Source: CAD feature listing. Evaluate the final solid. Frame: model axes, mm. A direction names the side the tool comes from. Round coordinates to 2 decimals unless told otherwise and drop trailing zeros. Order: outer loops, then holes, each group sorted by start corner. A loop starts at its lowest first (then second) coordinate and runs counter-clockwise, first axis right, second up. Notation, with made-up numbers: (-27.75, 1) -> (-16.75, 1) arc R23 cw to (-16.75, 22) -> close; hole circle Ø9 at (62, 32). An arc over 180 degrees is marked (long way). Answer as CSV lines item,"result".
from build123d import *

# Parameters (mm, degrees)
SKETCH1_R           = 1.5
BOSS_EXTRUDE1_DEPTH = 2
BOSS_EXTRUDE2_DEPTH = 38.1
BOSS_EXTRUDE3_DEPTH = 1.5
BOSS_EXTRUDE6_DEPTH = 27.94


with BuildPart() as part:
    # Sketch1 → Boss-Extrude1 (new body)
    with BuildSketch(Plane(origin=(0, 0, 0), x_dir=(1, 0, 0), z_dir=(0, 1, 0))):
        Polygon((-14, -7.1960018), (-3.6637, -7.1960018), (-3.6637, -14.7), (-1.6637, -14.7), (-1.6637, -2), (1.6637, -2), (1.6637, -14.7), (3.6637, -14.7), (3.6637, -7.1960018), (14, -7.1960018), (14, 5.5039982), (-14, 5.5039982), align=None)
        with Locations(Location((-11, -0.8460018, 0), (0, 0, 270))):
            Circle(SKETCH1_R, mode=Mode.SUBTRACT)
        with Locations(Location((11, -0.8460018, 0), (0, 0, 270))):
            Circle(SKETCH1_R, mode=Mode.SUBTRACT)
    extrude(amount=BOSS_EXTRUDE1_DEPTH)

    # Sketch1_3 → Boss-Extrude2 (add)
    with BuildSketch(Plane(origin=(0, 0, 0), x_dir=(1, 0, 0), z_dir=(0, 1, 0))):
        Polygon((3.6637, 0), (-3.6637, 0), (-3.6637, -7.1960018), (-3.6637, -14.7), (-1.6637, -14.7), (-1.6637, -2), (1.6637, -2), (1.6637, -14.7), (3.6637, -14.7), (3.6637, -7.1960018), align=None)
    extrude(amount=BOSS_EXTRUDE2_DEPTH)

    # Sketch2 → Boss-Extrude3 (add)
    with BuildSketch(Plane(origin=(0, 0, 7.1960018), x_dir=(-1, 0, 0), z_dir=(0, 0, -1))):
        Polygon((3.6637, 2), (3.6637, 33.75), (14, 2), align=None)
        Polygon((-14, 2), (-3.6637, 2), (-3.6637, 33.75), align=None)
    extrude(amount=BOSS_EXTRUDE3_DEPTH)

    # Sketch6 → Boss-Extrude6 (add)
    with BuildSketch(Plane(origin=(0, 38.1, 0), x_dir=(1, 0, 0), z_dir=(0, 1, 0))):
        Polygon((1.6637, -14.7), (3.6637, -14.7), (3.6637, 0), (-3.6637, 0), (-3.6637, -14.7), (-1.6637, -14.7), (-1.6637, -2), (1.6637, -2), align=None)
    extrude(amount=BOSS_EXTRUDE6_DEPTH)

    # Mirror6: part across plane


with BuildPart() as part_1:
    add(part.part)
    add(part.part.mirror(Plane(origin=(0, 66.04, 0), x_dir=(0, 0, 1), z_dir=(0, -1, 0))))


solid = part_1.part
1. Reachability of faces 4 (the flat face through (-8, 10, 7.196)), 5 (the flat face through (1.664, 67, 8)), 6 (the flat face through (3.664, 67, 7)), 7 (the flat face through (0, 67, 0)) from +Z, -Z, +X, -X, +Y, -Y: full face, straight path, thin tool, end or side. Return the list, or none.
Results below:
face 4,"+Z, -X, +Y, -Y"
face 5,"+Z, +Y, -Y"
face 6,"+X"
face 7,"-Z, +X, -X"
2. Section query D-D on z = 12.5. Return loops of the section in (x, y).
Results below:
outline,"(-3.66, 0) -> (-1.66, 0) -> (-1.66, 132.08) -> (-3.66, 132.08) -> close; (1.66, 0) -> (3.66, 0) -> (3.66, 132.08) -> (1.66, 132.08) -> close"
3. Section query A-A on z = -2.5. Return loops of the section in (x, y), and give its area (3 significant figures).
Results below:
outline,"(-14, 0) -> (14, 0) -> (14, 2) -> (-14, 2) -> close; (-14, 130.08) -> (14, 130.08) -> (14, 132.08) -> (-14, 132.08) -> close"
area,"112 mm2"
4. Mould query, pull axis Y, two halves, no side actions, for faces 1 (the flat face through (8.76, 113.98, 6.46)), 2 (the flat face through (0, 0, 0)), 3 (the flat face through (0, 67, 2)). Classes: released by +Y, released by -Y, zero draft, split by the parting line, or undercut.
Results below:
face 1,"undercut"
face 2,"released by -Y"
face 3,"zero draft"
5. Pin query (flat end, axial travel): pin 1 (3 mm diameter, centred on x = -11, y = 14, fed in from +Z); pin 2 (2.5 mm diameter, centred on x = 11, z = 0.85, fed in from -Y); pin 3 (4 mm diameter, centred on x = 4.5, z = 5, fed in from -Y); pin 4 (10 mm diameter, centred on y = 46, z = 1, fed in from +X). Return the tip coordinate at first contact, or that it passes through.
Results below:
pin 1,"z = 7.2"
pin 2,"through"
pin 3,"y = 0"
pin 4,"x = 3.66"
6. Section query B-B on y = 87. Return loops of the section in (x, z).
Results below:
outline,"(-3.66, 0) -> (3.66, 0) -> (3.66, 14.7) -> (1.66, 14.7) -> (1.66, 2) -> (-1.66, 2) -> (-1.66, 14.7) -> (-3.66, 14.7) -> close"
7. Section query C-C on x = -11. Return loops of the section in (y, z).
Results below:
outline,"(0, -5.5) -> (2, -5.5) -> (2, -0.65) -> (0, -0.65) -> close; (0, 2.35) -> (2, 2.35) -> (2, 5.7) -> (11.22, 5.7) -> (11.22, 7.2) -> (0, 7.2) -> close; (120.86, 5.7) -> (130.08, 5.7) -> (130.08, 2.35) -> (132.08, 2.35) -> (132.08, 7.2) -> (120.86, 7.2) -> close; (130.08, -5.5) -> (132.08, -5.5) -> (132.08, -0.65) -> (130.08, -0.65) -> close"
8. Line query: L1, parallel to X at y = 98.5, z = 10.75; L2, parallel to Y at x = -5.75, z = 3.5; L3, parallel to X at y = 17, z = 0.25. Output: solid intervals per line, ascending. Write a range as [from, to].
Results below:
L1,"[-3.66, -1.66], [1.66, 3.66]"
L2,"[0, 2], [130.08, 132.08]"
L3,"[-3.66, 3.66]"
